The drawing under review shows one solid part. Ordinate dimensions are in mm from its lowest x, y, z. Round coordinates to 2 decimals unless told otherwise and drop trailing zeros. Order: outer loops, then holes, each group sorted by start corner. A loop starts at its lowest first (then second) coordinate and runs counter-clockwise, first axis right, second up. Notation, with made-up numbers: (-29, 31) -> (5, 31) arc R19 cw to (5, 56) -> close; hole circle Ø6 at (-26.5, -40). An arc over 180 degrees is marked (long way). Put each result on its own line as item: value. Start each with the question number.
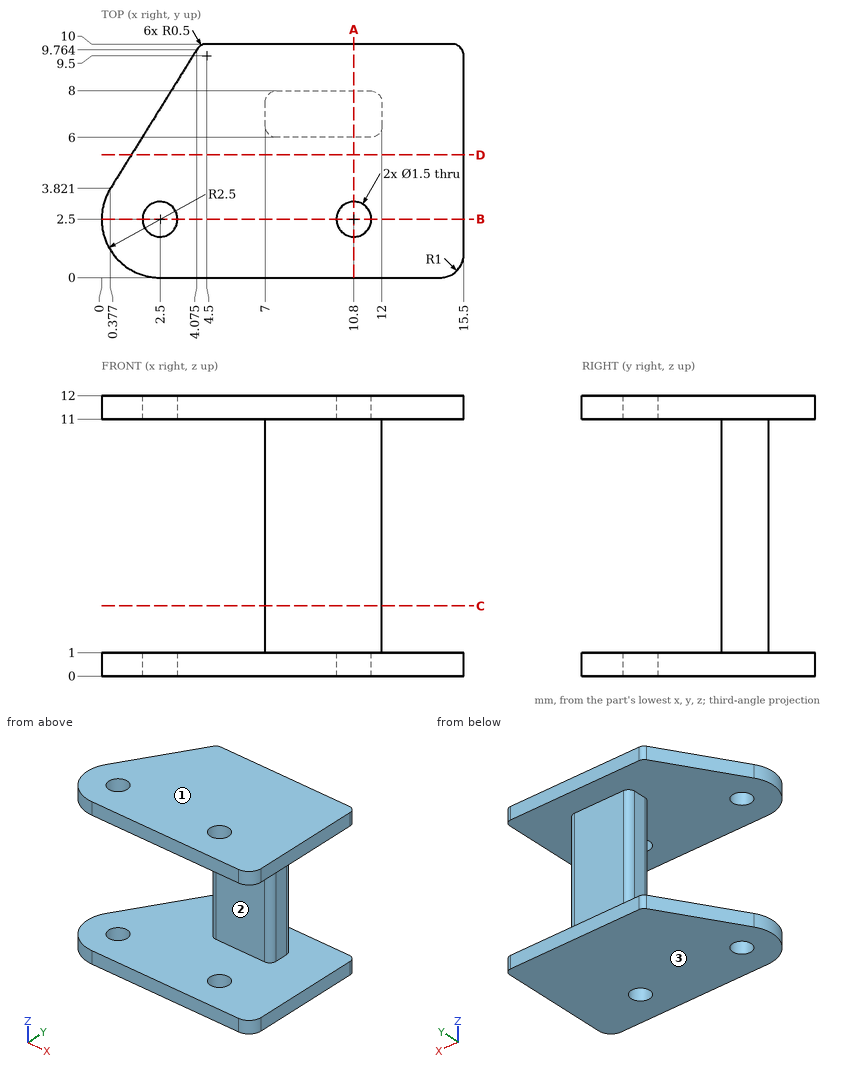
Item 1: Consider section B-B, the plane y = 2.5. Write out the cut boundary in (x, z).
Item 2: Insertion check: pin 1 Ø3 at (x, z) = (10, 8) entering from +Y; pin 2 Ø1.1 at (y, z) = (7, 3.5) entering from -X; pin 3 Ø1 at (y, z) = (7, 8) entering from +X. Each pin has a flat end and moves straight along its axis. Give the tip position at first contact, or say it passes through.
Item 3: Mouldability with a two-part tool opening along Z and no side actions: class the marked faces 1, 2 and 3 as +Z half, -Z half, draft (parallel to the pull), parting line (faces both ways), or undercut.
Item 4: Consider section D-D, the plane y = 5.25. Write out the cut boundary in (x, z).
Item 5: Consider section A-A, the plane x = 10.8. Write out the cut boundary in (y, z).
Item 6: Consider section C-C, the plane z = 3. Write out the cut boundary in (x, y).
Item 7: For L1, parallel to Z at x = 8, y = 9; L2, parallel to X at y = 2.75, z = 0.5; L3, parallel to Y at x = 10.8, z = 0.65, list the stretches that pass through material, from the lowest coordinate up.
Evaluation:
1. outline: (0, 0) -> (1.75, 0) -> (1.75, 1) -> (0, 1) -> close; (0, 11) -> (1.75, 11) -> (1.75, 12) -> (0, 12) -> close; (3.25, 0) -> (10.05, 0) -> (10.05, 1) -> (3.25, 1) -> close; (3.25, 11) -> (10.05, 11) -> (10.05, 12) -> (3.25, 12) -> close; (11.55, 0) -> (15.5, 0) -> (15.5, 1) -> (11.55, 1) -> close; (11.55, 11) -> (15.5, 11) -> (15.5, 12) -> (11.55, 12) -> close
2. pin 1: stops at y = 8
2. pin 2: stops at x = 7
2. pin 3: stops at x = 12
3. face 1: +Z half
3. face 2: undercut
3. face 3: -Z half
4. outline: (1.27, 0) -> (15.5, 0) -> (15.5, 1) -> (1.27, 1) -> close; (1.27, 11) -> (15.5, 11) -> (15.5, 12) -> (1.27, 12) -> close
5. outline: (0, 0) -> (1.75, 0) -> (1.75, 1) -> (0, 1) -> close; (0, 11) -> (1.75, 11) -> (1.75, 12) -> (0, 12) -> close; (3.25, 0) -> (10, 0) -> (10, 1) -> (8, 1) -> (8, 11) -> (10, 11) -> (10, 12) -> (3.25, 12) -> (3.25, 11) -> (6, 11) -> (6, 1) -> (3.25, 1) -> close
6. outline: (7, 6.5) arc R0.5 ccw to (7.5, 6) -> (11.5, 6) arc R0.5 ccw to (12, 6.5) -> (12, 7.5) arc R0.5 ccw to (11.5, 8) -> (7.5, 8) arc R0.5 ccw to (7, 7.5) -> close
7. L1: z = 0 to 1, 11 to 12
7. L2: x = 0.01 to 1.79, 3.21 to 10.09, 11.51 to 15.5
7. L3: y = 0 to 1.75, 3.25 to 10
